Solid Edge part; units mm, degrees
sketch "Sketch1" plane through (0, 0, 0) normal (0, 0, 1) x (1, 0, 0)
  line L0 (21, -14) -> (21, 15.5)
  arc A0 (21, 15.5) -> (15.5, 21) centre (15.5, 15.5) ccw
  line L1 (15.5, 21) -> (-14, 21)
  arc A1 (-19.5, 15.5) -> (-14, 21) centre (-14, 15.5) cw
  arc A2 (-15.5, 11.5) -> (-19.5, 15.5) centre (-15.5, 15.5) cw
  line L2 (0, 11.5) -> (-15.5, 11.5)
  line L3 (11.5, 0) -> (11.5, -15.5)
  arc A3 (11.5, -15.5) -> (15.5, -19.5) centre (15.5, -15.5) ccw
  arc A4 (15.5, -19.5) -> (21, -14) centre (15.5, -14) ccw
  arc A5 (0, 11.5) -> (11.5, 0) centre (0, 0) cw
extrude "Protrusion1" add sketch "Sketch1" along normal blind 4
sketch "Sketch2" plane through (0, 0, 0) normal (0, 0, 1) x (1, 0, 0)
  circle A0 centre (-15.5, 15.5) radius 1.625
  circle A1 centre (-4.25, 14) radius 1.625
  circle A2 centre (15.5, 15.5) radius 1.625
  circle A3 centre (15.5, -3.15) radius 1.625
  circle A4 centre (15.5, -15.5) radius 1.5438
extrude "Cutout1" cut sketch "Sketch2" along normal through all
sketch "Sketch3" plane through (0.75, 0.75, 4) normal (0, 0, 1) x (0, 1, 0)
  circle A0 centre (14.75, 16.25) radius 3
  line L0 (13.25, 2) -> (10.75, 2)
  line L1 (10.75, 8) -> (10.75, 2)
  line L2 (13.25, 8) -> (10.75, 8)
  arc A1 (13.25, 8) -> (13.25, 2) centre (13.25, 5) cw
  circle A2 centre (14.75, -14.75) radius 3
  circle A3 centre (-3.9, -14.75) radius 3
  circle A4 centre (-16.25, -14.75) radius 3
extrude "VaciadoExtruido_2" cut sketch "Sketch3" against normal blind 3
chamfer "Chaflán_1" distance 0.5 angle 45 11 edges at (8.1317, 8.1317, 4) (11.5, -7.75, 4) (12.6716, -18.3284, 4) (19.3891, -17.8891, 4) (21, 0.75, 4) (19.3891, 19.3891, 4) (0.75, 21, 4) (-17.8891, 19.3891, 4) (-18.3284, 12.6716, 4) (-11.375, 11.5, 4) (-0.625, 11.5, 4)
For this review, take the finished solid that the model builds, in its own axes (mm). A direction names the side the tool comes from. Give positions to 0.01 mm unless a question says otherwise; leave off trailing zeros. Write each loop counter-clockwise with the first axis right and the second up, starting at its lowest first coordinate (ties: lowest second). Pieces come first, ordered by that corner, then holes.
Item 1: Take a section at A-A (z = 2.4). Give the boundary of the cut face in (x, y), and give its area (3 significant figures).
Item 2: Take a section at D-D (y = -12). Give the boundary of the cut face in (x, z).
Item 3: Machinability: for faces 5 (the face through (18.43, -16.15, 2.52)), 6 (the face through (-4.2, 17, 2.5)), 7 (the face through (-9, 11.5, 2)), which of the approach directions +Z, -Z, +X, -X, +Y, -Y give a long, thin tool a straight path to every point of the face, cutting with its end or side? Answer none if there is none.
Item 4: Take a section at C-C (y = -3.15). Give the boundary of the cut face in (x, z) (3 decimals), and give its area (3 significant figures).
Item 5: Insertion check: P1, Ø5, axis at x = 15.5, y = 15.5, coming from the +Z side; P2, Ø0.8, axis at y = 12.5, z = 2.5, coming from the -X side; P3, Ø1.5, axis at y = 13.5, z = 0.5, coming from the -X side. Each pin has a flat end and moves straight along its axis. Give the tip position at first contact, or say it passes through.
Item 6: The part is to be moulded in two halves that separate along Y. For faces 1 (the face through (-14, 14, 1)), 2 (the face through (19.096, 19.176, 3.858)), 3 (the face through (16.25, 16.94, 0.49)), 4 (the face through (9, 10, 0)), say which applies: +Y half, -Y half, draft (parallel to the pull), parting line (faces both ways), or undercut.
Item 7: Take a section at B-B (x = -4.25). Give the boundary of the cut face in (y, z) (3 decimals).
Item 8: Wall thickness on probe 1 along Y at (x, z) = (15.5, 0.5) (3 decimals); probe 2 along Y at (x, z) = (15.5, 1.95); probe 3 along X at (y, z) = (13, 2.05): over which ranges is each line inside the solid? List them lowest first.
Established:
1. outline: (-19.5, 15.5) arc R4 ccw to (-15.5, 11.5) - (-7.25, 11.5) - (-7.25, 14) arc R3 cw to (-1.25, 14) - (-1.25, 11.5) - (0, 11.5) arc R11.5 cw to (11.5, 0) - (11.5, -15.5) arc R4 ccw to (15.5, -19.5) arc R5.5 ccw to (21, -14) - (21, 15.5) arc R5.5 ccw to (15.5, 21) - (-14, 21) arc R5.5 ccw to start; hole circle Ø6 at (-15.5, 15.5); hole circle Ø6 at (15.5, -15.5); hole circle Ø6 at (15.5, -3.15); hole circle Ø6 at (15.5, 15.5)
1. area: 539 mm2
2. outline: (11.5, 0) - (21, 0) - (21, 3.5) - (20.5, 4) - (12, 4) - (11.5, 3.5) - close
3. face 5: +Z
3. face 6: +Z, -Y
3. face 7: +Z, -Z, -X, -Y
4. outline: (11.5, 0) - (13.875, 0) - (13.875, 1) - (12.5, 1) - (12.5, 4) - (12, 4) - (11.5, 3.5) - close; (17.125, 0) - (21, 0) - (21, 3.5) - (20.5, 4) - (18.5, 4) - (18.5, 1) - (17.125, 1) - close
4. area: 16.5 mm2
5. P1: stops at z = 1
5. P2: stops at x = -18.54
5. P3: stops at x = -19.3
6. face 1: undercut
6. face 2: +Y half
6. face 3: undercut
6. face 4: draft
7. outline: (11.5, 0) - (12.375, 0) - (12.375, 1) - (11.5, 1) - close; (15.625, 0) - (21, 0) - (21, 3.5) - (20.5, 4) - (17, 4) - (17, 1) - (15.625, 1) - close
8. probe 1: y = -19.5 to -17.044, -13.956 to -4.775, -1.525 to 13.875, 17.125 to 21
8. probe 2: y = -19.5 to -18.5, -12.5 to -6.15, -0.15 to 12.5, 18.5 to 21
8. probe 3: x = -18.62 to -17.16, -13.84 to -7.25, -1.25 to 13.84, 17.16 to 21
